CAD build for the part. Positions are in the model's coordinates, mm. Face numbers are marked on the shaded views. A direction names the side the tool comes from. Round coordinates to 2 decimals unless told otherwise and drop trailing zeros. Order: outer loops, then holes, each group sorted by start corner. A loop starts at its lowest first (then second) coordinate and runs counter-clockwise, first axis right, second up. Notation, with made-up numbers: (-3, 9) -> (16, 9) arc R12 ccw to (16, 13) -> close; hole circle Ø11 at (6, 27.5). An arc over 180 degrees is marked (long way). Answer as CSV lines item,"result". Start each with the question number.
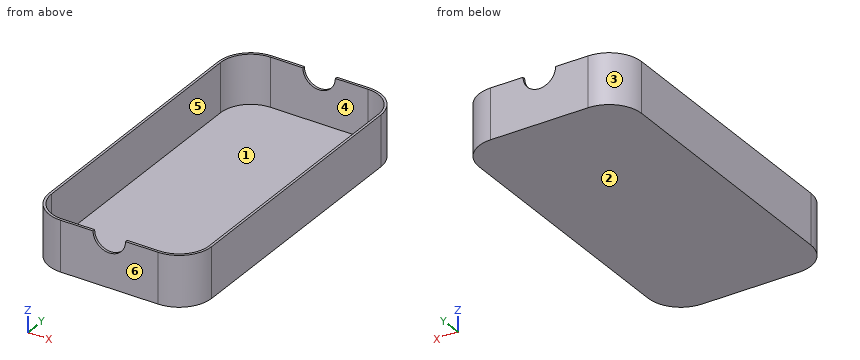
Autodesk Fusion 360 part; units mm, degrees
sketch "Sketch1" plane through (0, 0, 0) normal (0, 0, 1) x (1, 0, 0)
  line L0 (5, 0) -> (-55, 0)
  line L1 (-75, -20) -> (-75, -180)
  line L2 (-55, -200) -> (5, -200)
  line L3 (25, -180) -> (25, -20)
  arc A0 (25, -20) -> (5, 0) centre (5, -20) ccw
  arc A1 (-55, 0) -> (-75, -20) centre (-55, -20) ccw
  arc A2 (5, -200) -> (25, -180) centre (5, -180) ccw
  arc A3 (-75, -180) -> (-55, -200) centre (-55, -180) ccw
  dimension "d1" = 200
  dimension "d2" = 100
  dimension "d3" = 20
extrude "Extrude1" add sketch "Sketch1" along normal blind 1
sketch "Sketch2" plane through (0, 0, 1) normal (0, 0, 1) x (-1, 0, 0)
  arc A0 (75, 180) -> (55, 200) centre (55, 180) ccw
  line L0 (55, 200) -> (-5, 200)
  arc A1 (-5, 200) -> (-25, 180) centre (-5, 180) ccw
  line L1 (-25, 180) -> (-25, 20)
  arc A2 (-25, 20) -> (-5, 0) centre (-5, 20) ccw
  line L2 (-5, 0) -> (55, 0)
  arc A3 (55, 0) -> (75, 20) centre (55, 20) ccw
  line L3 (75, 20) -> (75, 180)
  line L4 (-5, 1.5) -> (55, 1.5)
  arc A4 (55, 1.5) -> (73.5, 20) centre (55, 20) ccw
  line L5 (73.5, 20) -> (73.5, 180)
  arc A5 (73.5, 180) -> (55, 198.5) centre (55, 180) ccw
  line L6 (55, 198.5) -> (-5, 198.5)
  arc A6 (-5, 198.5) -> (-23.5, 180) centre (-5, 180) ccw
  line L7 (-23.5, 180) -> (-23.5, 20)
  arc A7 (-23.5, 20) -> (-5, 1.5) centre (-5, 20) ccw
  dimension "d6" = -1.5
extrude "Extrude2" add sketch "Sketch2" along normal blind 30
sketch "Sketch3" plane through (0, 0, 0) normal (0, 1, 0) x (-1, 0, 0)
  line L0 (-5, 0) -> (55, 0)
  line L1 (55, 0) -> (55, 31)
  line L2 (55, 31) -> (-5, 31)
  line L3 (-5, 31) -> (-5, 0)
  circle A0 centre (25, 31) radius 10
  dimension "d9" = 20
extrude "Extrude3" cut sketch "Sketch3" against normal blind 10 contours L2 A0 picked at (23.7822, 27.8971)
sketch "Sketch4" plane through (0, -200, 0) normal (0, -1, 0) x (1, 0, 0)
  line L0 (-55, 0) -> (5, 0)
  line L1 (5, 0) -> (5, 31)
  line L2 (5, 31) -> (-55, 31)
  line L3 (-55, 31) -> (-55, 0)
  circle A0 centre (-25, 31) radius 10
  dimension "d12" = 20
extrude "Extrude4" cut sketch "Sketch4" against normal blind 10 contours L2 A0 picked at (-26.2178, 27.8971)
Item 1: Band-saw the part on D-D, the plane y = -101. Give the cut face in (x, z), and give its area (3 significant figures).
Item 2: Probe line 1 (X direction, y = -84.5, z = 21); line 2 (Y direction, x = -46, z = 9); line 3 (Z direction, x = -34, y = -100). List the from-to ranges inside material, lowest first.
Item 3: Pin check, flat tip, straight feed: pin 1 (5 mm diameter, centred on x = -60.5, z = 26, fed in from -Y). Stop position of the tip, or through.
Item 4: Band-saw the part on C-C, the plane z = 26.5. Give the cut face in (x, y), and give its area (3 significant figures).
Item 5: Band-saw the part on B-B, the plane x = -25. Give the cut face in (y, z).
Item 6: Mould opens along Y. For the marked faces 1, 2, 3 and 4 say: released by +Y, released by -Y, zero draft, split by the parting line, or undercut.
Item 7: Tool access for the marked faces 5 and 6: list every direction of +Z, -Z, +X, -X, +Y, -Y with a clear straight run to the whole face (end or side of a thin tool).
Item 8: Band-saw the part on A-A, the plane z = 9.5. Give the cut face in (x, y), and give its area (3 significant figures).
Values:
1,outline,"(-75, 0) -> (25, 0) -> (25, 31) -> (23.5, 31) -> (23.5, 1) -> (-73.5, 1) -> (-73.5, 31) -> (-75, 31) -> close"
1,area,"190 mm²"
2,line 1,"-75 to -73.5, 23.5 to 25"
2,line 2,"-200 to -198.5, -1.5 to 0"
2,line 3,"0 to 1"
3,pin 1,"y = -199.77"
4,outline,"(-75, -180) arc R20 ccw to (-55, -200) -> (-33.93, -200) -> (-33.93, -198.5) -> (-55, -198.5) arc R18.5 cw to (-73.5, -180) -> (-73.5, -20) arc R18.5 cw to (-55, -1.5) -> (-33.93, -1.5) -> (-33.93, 0) -> (-55, 0) arc R20 ccw to (-75, -20) -> close; (-16.07, -200) -> (5, -200) arc R20 ccw to (25, -180) -> (25, -20) arc R20 ccw to (5, 0) -> (-16.07, 0) -> (-16.07, -1.5) -> (5, -1.5) arc R18.5 cw to (23.5, -20) -> (23.5, -180) arc R18.5 cw to (5, -198.5) -> (-16.07, -198.5) -> close"
4,area,"788 mm²"
5,outline,"(-200, 0) -> (0, 0) -> (0, 21) -> (-1.5, 21) -> (-1.5, 1) -> (-198.5, 1) -> (-198.5, 21) -> (-200, 21) -> close"
6,face 1,"undercut"
6,face 2,"zero draft"
6,face 3,"released by +Y"
6,face 4,"undercut"
7,face 5,"+Z"
7,face 6,"+Z, -Z, +X, -X, -Y"
8,outline,"(-75, -180) arc R20 ccw to (-55, -200) -> (5, -200) arc R20 ccw to (25, -180) -> (25, -20) arc R20 ccw to (5, 0) -> (-55, 0) arc R20 ccw to (-75, -20) -> close; hole (-73.5, -180) arc R18.5 ccw to (-55, -198.5) -> (5, -198.5) arc R18.5 ccw to (23.5, -180) -> (23.5, -20) arc R18.5 ccw to (5, -1.5) -> (-55, -1.5) arc R18.5 ccw to (-73.5, -20) -> close"
8,area,"841 mm²"
